Verification items for the finished model (mm, model axes). Face numbers are marked on the shaded views. A direction names the side the tool comes from. Round coordinates to 2 decimals unless told otherwise and drop trailing zeros. Write each loop counter-clockwise with the first axis right and the second up, starting at its lowest first coordinate (ties: lowest second). Pieces come first, ordered by that corner, then holes. Notation, with made-up numbers: M 54.5,-35 L 102.5,-35 A22 cw 102.5,-9 Z; hole C -18.75,-32 d11. An arc over 180 degrees is marked long. One line per question, with ' | ' between items. Start each with the question number.
Q1. Thickness scan on line 1 along Z through (x, y) = (11.5, 16); line 2 along Y through (x, z) = (0, 5.75); line 3 along Y through (x, z) = (0, 16). Record the ranges inside material, lowest first. Write a range as from..to.
Q2. Cross-section at D-D (y = -10). Record the boundary of the cut face in (x, z).
Q3. Gauge pin test, flat ends, axial feed: pin 1 (6 mm diameter, centred on y = 2.5, z = 4, fed in from -X); pin 2 (1.5 mm diameter, centred on x = -11.5, z = 3, fed in from +Y); pin 3 (3 mm diameter, centred on x = 11, z = 6, fed in from +Y); pin 4 (10 mm diameter, centred on x = -12.5, y = 4.5, fed in from -Z). Record the tip position at first contact, or that the pin passes through.
Q4. Tool access check on the marked faces 4, 5 and 6. Record the directions out of +Z, -Z, +X, -X, +Y, -Y that give a thin tool (end or side, any length) a straight path to the whole face; none if there is none.
Q5. Cross-section at C-C (z = 1.5). Record the boundary of the cut face in (x, y), then the cut area to 3 significant figures.
Q6. Release check for a two-part mould opening along Y. For the marked faces 1, 2 and 3 record: released by +Y, released by -Y, zero draft, split by the parting line, or undercut.
Q7. Cross-section at A-A (x = 0). Record the boundary of the cut face in (y, z).
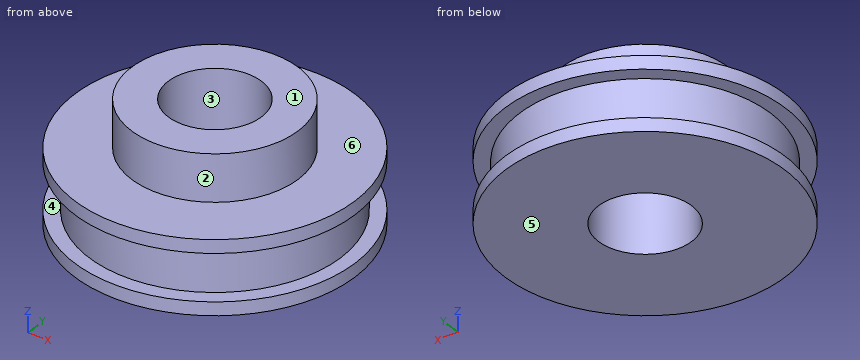
from build123d import *

# Parameters (mm, degrees)
SKETCH_1_R          = 21
EXTRUDE_1_DEPTH     = 2
SKETCH_2_R          = 18.85
EXTRUDE_2_DEPTH     = 7
SKETCH_3_R          = 21
EXTRUDE_3_DEPTH     = 2
SKETCH_4_R          = 12.5
EXTRUDE_4_DEPTH     = 7
SKETCH_5_R          = 7
CUT_EXTRUDE_1_DEPTH = 35.727510708


with BuildPart() as part:
    # 草图1 → 凸台-拉伸1 (new body)
    with BuildSketch(Plane.XY):
        Circle(SKETCH_1_R)
    extrude(amount=EXTRUDE_1_DEPTH)

    # 草图2 → 凸台-拉伸2 (add)
    with BuildSketch(Plane.XY.offset(2)):
        Circle(SKETCH_2_R)
    extrude(amount=EXTRUDE_2_DEPTH)

    # 草图3 → 凸台-拉伸3 (add)
    with BuildSketch(Plane.XY.offset(9)):
        Circle(SKETCH_3_R)
    extrude(amount=EXTRUDE_3_DEPTH)

    # 草图4 → 凸台-拉伸4 (add)
    with BuildSketch(Plane.XY.offset(11)):
        Circle(SKETCH_4_R)
    extrude(amount=EXTRUDE_4_DEPTH)

    # 草图5 → 切除-拉伸1 (cut, through all)
    with BuildSketch(Plane.XY.offset(18)):
        Circle(SKETCH_5_R)
    extrude(amount=-CUT_EXTRUDE_1_DEPTH, mode=Mode.SUBTRACT)


solid = part.part
Determined:
1) line 1: z = 0..2, 9..11 | line 2: y = -18.85..-7, 7..18.85 | line 3: y = -12.5..-7, 7..12.5
2) outline: M -18.47,0 L 18.47,0 L 18.47,2 L 15.98,2 L 15.98,9 L 18.47,9 L 18.47,11 L 7.5,11 L 7.5,18 L -7.5,18 L -7.5,11 L -18.47,11 L -18.47,9 L -15.98,9 L -15.98,2 L -18.47,2 Z
3) pin 1: stops at x = -21 | pin 2: stops at y = 15.48 | pin 3: stops at y = 16.28 | pin 4: stops at z = 0
4) face 4: none | face 5: -Z, +X, -X, +Y, -Y | face 6: +Z
5) outline: C 0,0 d42; hole C 0,0 d14 | area: 1,230 mm²
6) face 1: zero draft | face 2: split by the parting line | face 3: undercut
7) outline: M -21,0 L -7,0 L -7,18 L -12.5,18 L -12.5,11 L -21,11 L -21,9 L -18.85,9 L -18.85,2 L -21,2 Z; M 7,0 L 21,0 L 21,2 L 18.85,2 L 18.85,9 L 21,9 L 21,11 L 12.5,11 L 12.5,18 L 7,18 Z
